Verification items for this drawing (mm, ordinates from the low corner). A direction names the side the tool comes from. Round coordinates to 2 decimals unless told otherwise and drop trailing zeros. Loops run counter-clockwise (first coordinate to the right, second up) from the corner with the lowest first, then second, coordinate; pieces in that order, holes last. Notation, with made-up numbers: (-1.5, -26.5) -> (37.5, -26.5) arc R34 cw to (37.5, 9.5) -> close; hole circle Ø2 at (19, -23). An arc over 180 degrees is marked (long way). Use a Markdown table: item, result. Add a question column.
Q1. Sectioned sample at B-B, the plane x = 6.5. Enter the section's corners in (y, z).
Q2. Sectioned sample at D-D, the plane x = 11. Enter the section's corners in (y, z), then the cut area to 3 significant figures.
Q3. Set-up check for the marked faces 1 and 2: record each of +Z, -Z, +X, -X, +Y, -Y from which the full face is reachable in a straight line by a thin tool's end or side.
Q4. Sectioned sample at A-A, the plane z = 11. Enter the section's corners in (x, y).
Q5. Material ranges on L1, parallel to Y at x = 3.5, z = 12.75; L2, parallel to Z at x = 10, y = 2.9; L3, parallel to Z at x = 9, y = 0.9, recorded low to high.
Q6. Gauge pin test, flat ends, axial feed: P1, Ø1.5, axis at x = 9, z = 18.5, coming from the +Y side; P2, Ø1, axis at x = 7, y = 2, coming from the -Z side. Record the tip position at first contact, or that the pin passes through.
Q7. Sectioned sample at C-C, the plane y = 3.75. Enter the section's corners in (x, z), then the cut area to 3 significant figures.
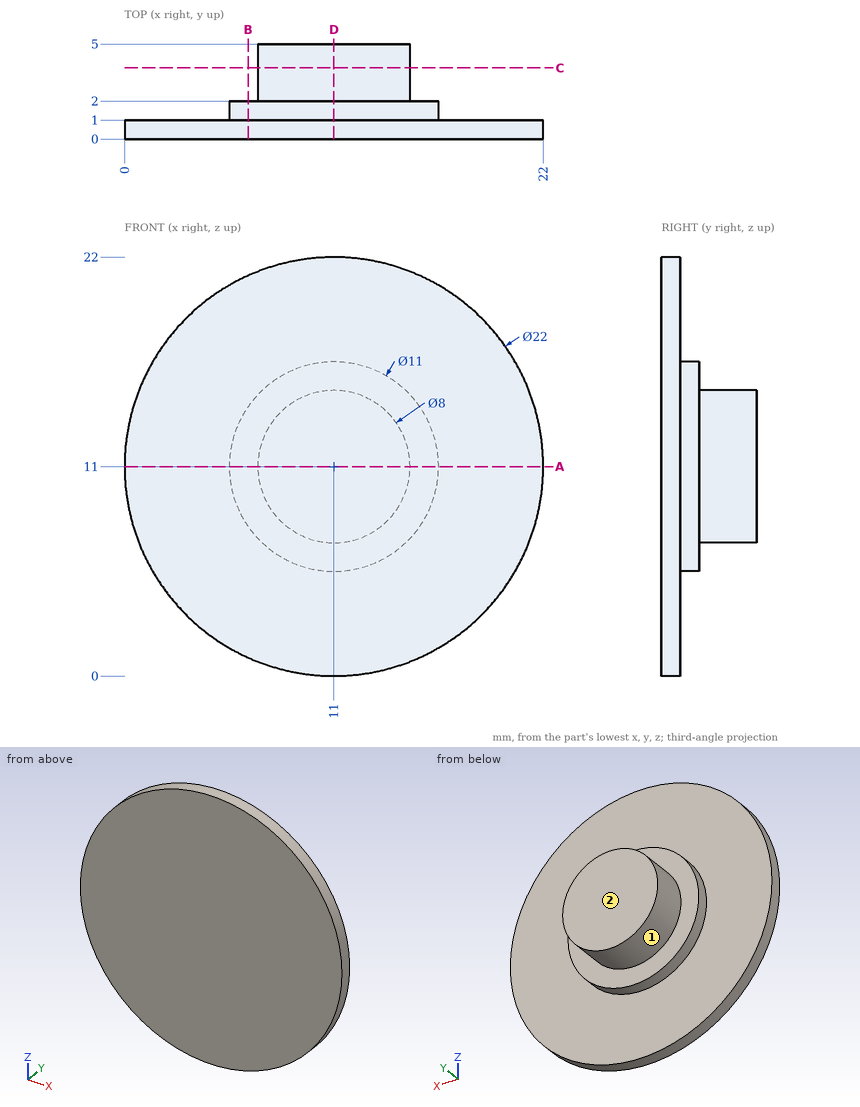
Values:
| question | item | result |
|---|---|---|
| 1 | outline | (0, 0.96) -> (1, 0.96) -> (1, 7.84) -> (2, 7.84) -> (2, 14.16) -> (1, 14.16) -> (1, 21.04) -> (0, 21.04) -> close |
| 2 | outline | (0, 0) -> (1, 0) -> (1, 5.5) -> (2, 5.5) -> (2, 7) -> (5, 7) -> (5, 15) -> (2, 15) -> (2, 16.5) -> (1, 16.5) -> (1, 22) -> (0, 22) -> close |
| 2 | area | 57.0 mm^2 |
| 3 | face 1 | +Y |
| 3 | face 2 | +Z, -Z, +X, -X, +Y |
| 4 | outline | (0, 0) -> (22, 0) -> (22, 1) -> (16.5, 1) -> (16.5, 2) -> (15, 2) -> (15, 5) -> (7, 5) -> (7, 2) -> (5.5, 2) -> (5.5, 1) -> (0, 1) -> close |
| 5 | L1 | 0 to 1 |
| 5 | L2 | 7.13 to 14.87 |
| 5 | L3 | 0.18 to 21.82 |
| 6 | P1 | y = 1 |
| 6 | P2 | z = 6.76 |
| 7 | outline | circle Ø8 at (11, 11) |
| 7 | area | 50.3 mm^2 |
